from build123d import *

# Parameters (mm, degrees)
F0_R     = 9
F0_R_2   = 5.4
F1_DEPTH = 30
F2_DEPTH = 5
F4_DEPTH = 2
F5_DEPTH = 30
F6_R     = 1


with BuildPart() as f1:
    # F0 (on Top) → F1 (new body)
    with BuildSketch(Plane.XY):
        Circle(F0_R)
        Circle(F0_R_2, mode=Mode.SUBTRACT)
    extrude(amount=F1_DEPTH)

    # F0 (on Top) → F2 (join)
    with BuildSketch(Plane.XY):
        Circle(F0_R_2)
    extrude(amount=F2_DEPTH)

    # F3 (on face) → F4 (join)
    with BuildSketch(Plane.XY.offset(30)):
        with BuildLine():
            Line((0, 11), (0, 13))
            ThreePointArc((0, 13), (-13, 0), (0, -13))
            Line((0, -13), (0, -11))
            ThreePointArc((0, -11), (-11, 0), (0, 11))
        make_face()
        with BuildLine():
            Line((0, 9), (0, 11))
            ThreePointArc((0, 11), (-11, 0), (0, -11))
            Line((0, -11), (0, -9))
            ThreePointArc((0, -9), (-9, 0), (0, 9))
        make_face()
    extrude(amount=-F4_DEPTH)

    # F3 (on face) → F5 (join)
    with BuildSketch(Plane.XY.offset(30)):
        with BuildLine():
            Line((0, 11), (0, 13))
            ThreePointArc((0, 13), (-13, 0), (0, -13))
            Line((0, -13), (0, -11))
            ThreePointArc((0, -11), (-11, 0), (0, 11))
        make_face()
    extrude(amount=-F5_DEPTH)

    # F6
    f6_edges = [f1.edges().sort_by_distance(p)[0] for p in [
        (-9, 0, 0),
        (-13, 0, 0),
        (-13, 0, 30),
        (0, 13, 15),
        (0, -13, 15),
        (0, -11, 30),
        (0, 11, 30),
        (6.363961, -6.363961, 30),
        (6.363961, 6.363961, 30),
        (-5.4, 0, 30),
    ]]
    fillet(f6_edges, radius=F6_R)


solid = f1.part
Model file for the job. Use its own axes, mm. A direction names the side the tool comes from. Round coordinates to 2 decimals unless told otherwise and drop trailing zeros. Loops run counter-clockwise (first coordinate to the right, second up) from the corner with the lowest first, then second, coordinate; pieces in that order, holes last. Notation, with made-up numbers: M -12,85 L 46,85 A36 ccw 46,119 Z; hole C 13,69.25 d1. An arc over 180 degrees is marked long. One line per question, with ' | ' between items.
1) Band-saw the part on B-B (y = 0). Give the cut face in (x, z).
Solved:
outline: M -13,1 A1 ccw -12,0 L -11,0 L -11,28 L -9,28 L -9,1 A1 ccw -8,0 L 8,0 A1 ccw 9,1 L 9,29 A1 ccw 8,30 L 6.4,30 A1 ccw 5.4,29 L 5.4,5 L -5.4,5 L -5.4,29 A1 ccw -6.4,30 L -12,30 A1 ccw -13,29 Z
2) 3-axis set-ups, long thin cutter, end or side, ignore diameter. For faces 4 (the cylindrical face through (-0.301, 10.423, 29.715)), 5 (the cylindrical face through (-1.17, -5.27, 16.83)), 6 (the cylindrical face through (-0.301, -10.366, 29.715)): which of +Z, -Z, +X, -X, +Y, -Y reach the whole face in a straight line?
Solved:
face 4: +Z, +X, +Y | face 5: +Z | face 6: +Z, +X, -Y
3) Drill centre lines: line 1 along X through (y, z) = (-0.25, 14); line 2 along X through (y, z) = (1.75, 23); line 3 along Y through (x, z) = (-6.75, 12). Where is each one in solid material? Low to high.
Solved:
line 1: x = -13 to -11, -9 to -5.39, 5.39 to 9 | line 2: x = -12.88 to -10.86, -8.83 to -5.11, 5.11 to 8.83 | line 3: y = -11.11 to -8.69, -5.95 to 5.95, 8.69 to 11.11
4) Mould opens along X. For faces 1 (the flat face through (-7, 0, 30)), 2 (the flat face through (0, -11.5, 15.6)), 3 (the flat face through (-9.2, 0.1, 28)) say: +X half, -X half, draft (parallel to the pull), parting line (faces both ways), or undercut.
Solved:
face 1: draft | face 2: +X half | face 3: undercut
5) Flat gauge pins, fed straight in: pin 1 (8 mm diameter, centred on y = 9, z = 7, fed in from -X); pin 2 (8.5 mm diameter, centred on x = 0, y = 0, fed in from +Z); pin 3 (5 mm diameter, centred on x = 3.5, z = 23, fed in from -Y). Where does each tip first touch, or does it go through?
Solved:
pin 1: stops at x = -12 | pin 2: stops at z = 5 | pin 3: stops at y = -8.94
6) Band-saw the part on A-A (z = 21). Give the cut face in (x, y), then the cut area to 3 significant figures.
Solved:
outline: C 0,0 d18; M -1.08,-12.95 A1 ccw 0,-11.96 L 0,-11 A11 cw 0,11 L 0,11.96 A1 ccw -1.08,12.95 A13 ccw Z; hole C 0,0 d10.8 | area: 238 mm²
